Verification items for the finished model (mm, model axes). Face numbers are marked on the shaded views. A direction names the side the tool comes from. Coordinates: 2 decimals unless noted, no trailing zeros. Order: outer loops, then holes, each group sorted by start corner. A loop starts at its lowest first (then second) coordinate and runs counter-clockwise, first axis right, second up. Notation, with made-up numbers: (-20.5, -38.75) -> (24.5, -38.75) arc R19 cw to (24.5, -30.75) -> close; hole circle Ø10 at (-20.75, 86.5). An arc over 180 degrees is marked (long way). Write item = value, one per line. Start each with the question number.
from build123d import *

# Parameters (mm, degrees)
ESQUISSE1_W             = 17
ESQUISSE1_H             = 59
BOSS_EXTRU_1_DEPTH      = 2
ESQUISSE2_W             = 8.5
ESQUISSE2_H             = 59
BOSS_EXTRU_2_DEPTH      = 6
ESQUISSE3_W             = 1.5
ESQUISSE3_H             = 23
ESQUISSE3_H_2           = 14
ENL_V_MAT_EXTRU_1_DEPTH = 6
ESQUISSE4_R             = 2.25
ENL_V_MAT_EXTRU_4_DEPTH = 22
ESQUISSE6_R             = 3.75
ENL_V_MAT_EXTRU_5_DEPTH = 6


with BuildPart() as part:
    # Esquisse1 → Boss.-Extru.1 (new body)
    with BuildSketch(Plane.XY):
        with Locations((8.5, -29.5)):
            Rectangle(ESQUISSE1_W, ESQUISSE1_H)
    extrude(amount=BOSS_EXTRU_1_DEPTH)

    # Esquisse2 → Boss.-Extru.2 (add)
    with BuildSketch(Plane.XY.offset(2)):
        with Locations((4.25, -29.5)):
            Rectangle(ESQUISSE2_W, ESQUISSE2_H)
    extrude(amount=BOSS_EXTRU_2_DEPTH)

    # Esquisse3 → Enlèv. mat.-Extru.1 (cut)
    with BuildSketch(Plane.XY.offset(8)):
        with Locations((2.75, -47.5)):
            Rectangle(ESQUISSE3_W, ESQUISSE3_H)
        with BuildLine():
            ThreePointArc((3.5, -33.702199257), (2.408191843, -34.627967907), (2, -36))
            Line((2, -36), (3.5, -36))
            Line((3.5, -36), (3.5, -33.702199257))
        make_face()
        with BuildLine():
            Line((3.5, -33.702199257), (3.5, -36))
            ThreePointArc((3.5, -36), (4.509962751, -34.990037249), (5.519925502, -36))
            Line((5.519925502, -36), (5.519925502, -33.702199257))
            ThreePointArc((5.519925502, -33.702199257), (4.509962751, -33.490037249), (3.5, -33.702199257))
        make_face()
        with BuildLine():
            Line((5.519925502, -33.702199257), (5.519925502, -36))
            Line((5.519925502, -36), (7.019925502, -36))
            ThreePointArc((7.019925502, -36), (6.611733659, -34.627967907), (5.519925502, -33.702199257))
        make_face()
        with Locations((6.269925502, -43)):
            Rectangle(ESQUISSE3_W, ESQUISSE3_H_2)
        with Locations((6.269925502, -16)):
            Rectangle(ESQUISSE3_W, ESQUISSE3_H_2)
        with Locations((2.75, -11.5)):
            Rectangle(ESQUISSE3_W, ESQUISSE3_H)
        with BuildLine():
            Line((3.5, -23), (2, -23))
            ThreePointArc((2, -23), (2.408191843, -24.372032093), (3.5, -25.297800743))
            Line((3.5, -25.297800743), (3.5, -23))
        make_face()
        with BuildLine():
            ThreePointArc((5.519925502, -23), (4.509962751, -24.009962751), (3.5, -23))
            Line((3.5, -23), (3.5, -25.297800743))
            ThreePointArc((3.5, -25.297800743), (4.509962751, -25.509962751), (5.519925502, -25.297800743))
            Line((5.519925502, -25.297800743), (5.519925502, -23))
        make_face()
        with BuildLine():
            Line((7.019925502, -23), (5.519925502, -23))
            Line((5.519925502, -23), (5.519925502, -25.297800743))
            ThreePointArc((5.519925502, -25.297800743), (6.611733659, -24.372032093), (7.019925502, -23))
        make_face()
    extrude(amount=-ENL_V_MAT_EXTRU_1_DEPTH, mode=Mode.SUBTRACT)

    # Esquisse4 → Enlèv. mat.-Extru.4 (cut)
    with BuildSketch(Plane.XY.offset(8)):
        with Locations((8.5, -29.5)):
            Circle(ESQUISSE4_R)
        with Locations((8.5, -54)):
            Circle(ESQUISSE4_R)
        with Locations((8.5, -5)):
            Circle(ESQUISSE4_R)
    extrude(amount=-ENL_V_MAT_EXTRU_4_DEPTH, mode=Mode.SUBTRACT)

    # Esquisse6 → Enlèv. mat.-Extru.5 (cut)
    with BuildSketch(Plane.XY.offset(8)):
        with Locations((8.5, -29.5)):
            Circle(ESQUISSE6_R)
        with Locations((8.5, -5)):
            Circle(ESQUISSE6_R)
        with Locations((8.5, -54)):
            Circle(ESQUISSE6_R)
    extrude(amount=-ENL_V_MAT_EXTRU_5_DEPTH, mode=Mode.SUBTRACT)


solid = part.part
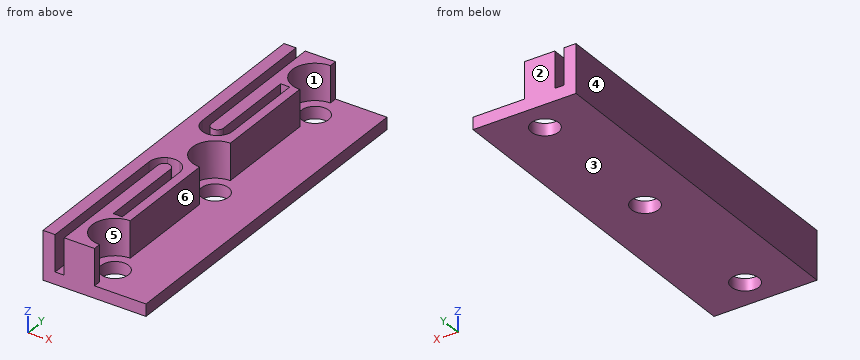
Item 1: Section check B-B (x = 10). Record the boundary of the cut face in (y, z), then the cut area to 3 significant figures.
Item 2: Gauge pin test, flat end, axial feed: P1, Ø1.8, axis at y = -43.5, z = 4.5, coming from the +X side. Record the tip position at first contact, or that the pin passes through.
Item 3: Tool access check on the marked faces 4, 5 and 6. Record the directions out of +Z, -Z, +X, -X, +Y, -Y that give a thin tool (end or side, any length) a straight path to the whole face; none if there is none.
Item 4: Section check C-C (y = -42.5). Record the boundary of the cut face in (x, z).
Item 5: Thickness scan on line 1 (X direction, y = -40, z = 3); line 2 (Y direction, x = 8.5, z = 0.75); line 3 (X direction, y = -54, z = 0.9). Record the ranges inside material, lowest first.
Item 6: Section check D-D (x = 13.75). Record the boundary of the cut face in (y, z), then the cut area to 3 significant figures.
Item 7: Mould release check, pull along Y, two halves, no side actions. Record for the marked faces 1, 2 and 3: pulls with the +Y half, pulls with the -Y half, needs draft (parallel to the pull), parting line crosses it, or undercut.
Item 8: Section check A-A (y = -29.5). Record the boundary of the cut face in (x, z), then the cut area to 3 significant figures.
Filled sheet:
q1.outline = (-59, 0) -> (-55.68, 0) -> (-55.68, 2) -> (-59, 2) -> close; (-52.32, 0) -> (-31.18, 0) -> (-31.18, 2) -> (-52.32, 2) -> close; (-27.82, 0) -> (-6.68, 0) -> (-6.68, 2) -> (-27.82, 2) -> close; (-3.32, 0) -> (0, 0) -> (0, 2) -> (-3.32, 2) -> close
q1.area = 97.9 mm^2
q2.P1 = 8.5
q3.face_4 = +Z, -Z, -X, +Y, -Y
q3.face_5 = +Z, +X
q3.face_6 = +Z, +X, +Y, -Y
q4.outline = (0, 0) -> (17, 0) -> (17, 2) -> (8.5, 2) -> (8.5, 8) -> (7.02, 8) -> (7.02, 2) -> (5.52, 2) -> (5.52, 8) -> (3.5, 8) -> (3.5, 2) -> (2, 2) -> (2, 8) -> (0, 8) -> close
q5.line_1 = 0 to 2, 3.5 to 5.52, 7.02 to 8.5
q5.line_2 = -59 to -56.25, -51.75 to -31.75, -27.25 to -7.25, -2.75 to 0
q5.line_3 = 0 to 6.25, 10.75 to 17
q6.outline = (-59, 0) -> (0, 0) -> (0, 2) -> (-59, 2) -> close
q6.area = 118 mm^2
q7.face_1 = undercut
q7.face_2 = pulls with the +Y half
q7.face_3 = needs draft
q8.outline = (0, 0) -> (6.25, 0) -> (6.25, 2) -> (4.75, 2) -> (4.75, 8) -> (0, 8) -> close; (10.75, 0) -> (17, 0) -> (17, 2) -> (10.75, 2) -> close
q8.area = 53.5 mm^2
